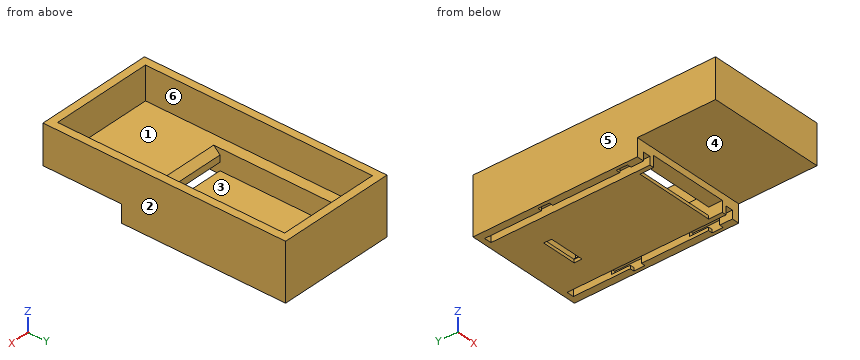
```python
from build123d import *

# Parameters (mm, degrees)
SKETCH4_W           = 29.99999933
SKETCH4_H           = 41.999999434
BOSS_EXTRUDE2_DEPTH = 4.499999806
SKETCH5_W           = 1.862979494
SKETCH5_H           = 40.647998452
CUT_EXTRUDE1_DEPTH  = 2.068
SKETCH2_W           = 1.025000587
SKETCH2_H           = 2.855999861
SKETCH2_H_2         = 2.855997533
CUT_EXTRUDE2_DEPTH  = 2.068
SKETCH3_W           = 1.025000587
SKETCH3_H           = 7.699999958
SKETCH3_H_2         = 7.699999959
CUT_EXTRUDE3_DEPTH  = 1.251
SKETCH6_W           = 8.999999612
SKETCH6_H           = 2.000000328
CUT_EXTRUDE4_DEPTH  = 1
SKETCH7_W           = 20.324639976
SKETCH7_H           = 3.493499942
CUT_EXTRUDE6_DEPTH  = 2.81
CUT_EXTRUDE7_DEPTH  = 3.699999806
SKETCH9_W           = 29.99999933
SKETCH9_H           = 61.999998987
SKETCH9_W_2         = 20.324639976
SKETCH9_H_2         = 36.506499492
BOSS_EXTRUDE3_DEPTH = 10
SKETCH10_W          = 25.99999933
SKETCH10_H          = 57.999998987
CUT_EXTRUDE8_DEPTH  = 8.4
CHAMFER1_SIZE       = 1.6


# Read off the part's stored shape, not the designer's step: Surface-Imported1
with BuildPart() as part:
    # Sketch4 → Boss-Extrude2 (new body)
    with BuildSketch(Plane.XY):
        with Locations((0, 20.999999717)):
            Rectangle(SKETCH4_W, SKETCH4_H)
    extrude(amount=BOSS_EXTRUDE2_DEPTH)

    # Sketch5 → Cut-Extrude1 (cut)
    with BuildSketch(Plane.XY):
        with Locations((-12.198510114, 20.323999226)):
            Rectangle(SKETCH5_W, SKETCH5_H)
        with Locations((12.198510114, 20.323999226)):
            Rectangle(SKETCH5_W, SKETCH5_H)
    extrude(amount=CUT_EXTRUDE1_DEPTH, mode=Mode.SUBTRACT)

    # Sketch2 → Cut-Extrude2 (cut)
    with BuildSketch(Plane.XY):
        with Locations((13.642500155, 4.677999998)):
            Rectangle(SKETCH2_W, SKETCH2_H)
        with Locations((13.642500155, 24.677999318)):
            Rectangle(SKETCH2_W, SKETCH2_H_2)
    extrude(amount=CUT_EXTRUDE2_DEPTH, mode=Mode.SUBTRACT)

    # Sketch3 → Cut-Extrude3 (cut)
    with BuildSketch(Plane.XY.offset(0.816999993)):
        with Locations((13.642500155, 7.100000046)):
            Rectangle(SKETCH3_W, SKETCH3_H)
        with Locations((13.642500155, 27.100000531)):
            Rectangle(SKETCH3_W, SKETCH3_H_2)
    extrude(amount=CUT_EXTRUDE3_DEPTH, mode=Mode.SUBTRACT)

    # Sketch6 → Cut-Extrude4 (cut)
    with BuildSketch(Plane.XY):
        with Locations((0, 31.999999657)):
            Rectangle(SKETCH6_W, SKETCH6_H)
    extrude(amount=CUT_EXTRUDE4_DEPTH, mode=Mode.SUBTRACT)

    # Sketch7 → Cut-Extrude6 (cut)
    with BuildSketch(Plane.XY):
        with Locations((0, 1.746749971)):
            Rectangle(SKETCH7_W, SKETCH7_H)
    extrude(amount=CUT_EXTRUDE6_DEPTH, mode=Mode.SUBTRACT)

    # Sketch8 → Cut-Extrude7 (cut)
    with BuildSketch(Plane.XY.offset(4.499999806)):
        Polygon((-9.362319988, 3.493499942), (-10.162319988, 3.493499942), (-10.162319988, 39.999999434), (10.162319988, 39.999999434), (10.162319988, 3.493499942), (9.362319988, 3.493499942), align=None)
    extrude(amount=-CUT_EXTRUDE7_DEPTH, mode=Mode.SUBTRACT)

    # Sketch9 → Boss-Extrude3 (add)
    with BuildSketch(Plane.XY.offset(4.499999806)):
        with Locations((0, 10.999999941)):
            Rectangle(SKETCH9_W, SKETCH9_H)
        with Locations((0, 21.746749688)):
            Rectangle(SKETCH9_W_2, SKETCH9_H_2, mode=Mode.SUBTRACT)
    extrude(amount=BOSS_EXTRUDE3_DEPTH)

    # Sketch10 → Cut-Extrude8 (cut)
    with BuildSketch(Plane.XY.offset(14.499999806)):
        with Locations((0, 10.999999941)):
            Rectangle(SKETCH10_W, SKETCH10_H)
    extrude(amount=-CUT_EXTRUDE8_DEPTH, mode=Mode.SUBTRACT)

    # Chamfer1
    chamfer1_edges = [part.edges().sort_by_distance(p)[0] for p in [
        (0, 3.493499942, 6.099999806),
    ]]
    chamfer(chamfer1_edges, length=CHAMFER1_SIZE)


with BuildPart() as body_2:
    # Split1: the piece on the far side of the plane
    add(part.part)
    split(bisect_by=Plane(origin=(0, 0, 0), x_dir=(0, 0, 1), z_dir=(1, 0, 0)), keep=Keep.BOTTOM)


with BuildPart() as part_1:
    add(part.part)

    # Split1
    split(bisect_by=Plane(origin=(0, 0, 0), x_dir=(0, 0, 1), z_dir=(1, 0, 0)), keep=Keep.TOP)

    # Mirror1: part across plane


with BuildPart() as part_2:
    add(part_1.part)
    add(part_1.part.mirror(Plane(origin=(0, 0, 0), x_dir=(0, 0, 1), z_dir=(1, 0, 0))))


solid = part_2.part
```
Work out the finished part from the listing and answer in its coordinate system (mm). Face numbers are marked on the shaded views. A direction names the side the tool comes from. Coordinates: 2 decimals unless noted, no trailing zeros. Order: outer loops, then holes, each group sorted by start corner. A loop starts at its lowest first (then second) coordinate and runs counter-clockwise, first axis right, second up. Notation, with made-up numbers: (61, 56) - (115, 56) arc R7 ccw to (115, 64) - close; hole circle Ø7 at (-38, 9). An arc over 180 degrees is marked (long way). Answer as a JSON object with one key per item and string values.
1. Find section D-D on z = 3.5. Determine the outline of the cut face in (x, y), plus the area to 3 significant figures.
Output values:
{"outline": "(-15, 0) - (15, 0) - (15, 42) - (-15, 42) - close; hole (-10.16, 3.49) - (10.16, 3.49) - (10.16, 40) - (-10.16, 40) - close", "area": "518 mm²"}
2. Consider line 1 (Y direction, x = -12.75, z = 10.5); line 2 (X direction, y = -3, z = 13.5); line 3 (Y direction, x = 9.5, z = 3.5). Determine where each line is inside the solid, lowest interval first.
Output values:
{"line 1": "y = -20 to -18, 40 to 42", "line 2": "x = -15 to -13, 13 to 15", "line 3": "y = 0 to 3.49, 40 to 42"}
3. Find section C-C on y = 15.5. Determine the outline of the cut face in (x, z).
Output values:
{"outline": "(-15, 0) - (-13.13, 0) - (-13.13, 2.07) - (-11.27, 2.07) - (-11.27, 0) - (11.27, 0) - (11.27, 2.07) - (13.13, 2.07) - (13.13, 0) - (15, 0) - (15, 14.5) - (13, 14.5) - (13, 6.1) - (10.16, 6.1) - (10.16, 0.8) - (-10.16, 0.8) - (-10.16, 6.1) - (-13, 6.1) - (-13, 14.5) - (-15, 14.5) - close"}
4. A tool of negligible diameter and unlimited length cuts with its end or side. For the marked faces 1, 2 and 3, from which of +Z, -Z, +X, -X, +Y, -Y can it reach the whole face along a straight path? Write none if from no direction.
Output values:
{"face 1": "+Z", "face 2": "+Z, -Z, +X, +Y, -Y", "face 3": "+Z, -Y"}
5. Find section A-A on x = 7.75. Determine the outline of the cut face in (y, z).
Output values:
{"outline": "(-20, 4.5) - (0, 4.5) - (0, 2.81) - (3.49, 2.81) - (3.49, 4.5) - (1.89, 6.1) - (-18, 6.1) - (-18, 14.5) - (-20, 14.5) - close; (3.49, 0) - (42, 0) - (42, 14.5) - (40, 14.5) - (40, 0.8) - (3.49, 0.8) - close"}
6. The mould has two halves that part along X. Classify the marked faces 4, 5 and 6: +X half, -X half, draft (parallel to the pull), parting line (faces both ways), or undercut.
Output values:
{"face 4": "draft", "face 5": "-X half", "face 6": "undercut"}
7. Find section B-B on z = 10.5. Determine the outline of the cut face in (x, y), plus the area to 3 significant figures.
Output values:
{"outline": "(-15, -20) - (15, -20) - (15, 42) - (-15, 42) - close; hole (-13, -18) - (13, -18) - (13, 40) - (-13, 40) - close", "area": "352 mm²"}
8. Each of these flat-tipped pins is pushed along its axis until it touches: P1, Ø1.1, axis at x = 13.5, z = 1, coming from the -Y side; P2, Ø0.6, axis at x = -12.5, z = 1.5, coming from the -Y side. Where does it stop, or does it pass through?
Output values:
{"P1": "stops at y = 0", "P2": "stops at y = 40.65"}
